Geometry: final body of the model. Coordinates: model frame, mm. Face numbers are marked on the shaded views. A direction names the side the tool comes from. Coordinates: 2 decimals unless noted, no trailing zeros. Loops run counter-clockwise (first coordinate to the right, second up) from the corner with the lowest first, then second, coordinate; pieces in that order, holes last. Notation, with made-up numbers: (5, -6.5) -> (55, -6.5) arc R18 ccw to (55, 17.5) -> close; hole circle Ø10 at (-19, 61.25). An arc over 180 degrees is marked (long way). One line per item, written item: value. Start each with the question number.
Item 1: Section query A-A on z = 0. Return loops of the section in (x, y), then the cut area to 3 significant figures.
Item 2: Contact query for flat-ended pins moving along their axis: pin 1 Ø2.5 at (x, z) = (60, 0) entering from +Y; pin 2 Ø3 at (x, z) = (45, 2) entering from -Y; pin 3 Ø1.5 at (y, z) = (1, -1.5) entering from +X. Output: stop coordinate, or through.
Item 3: Section query D-D on x = 48.5. Return loops of the section in (y, z), then the cut area to 3 significant figures.
Item 4: Section query C-C on y = 6.25. Return loops of the section in (x, z).
Item 5: Ray query, probe 1 along X at (y, z) = (2.75, 0); probe 2 along Y at (x, z) = (34, 1.15); probe 3 along X at (y, z) = (5.5, 0). Return the intervals inside material, ascending. Write a range as from..to.
Item 6: Section query B-B on y = 3.25. Return loops of the section in (x, z).
Item 7: Set-up query: the marked faces 1 and 2. Return all of +Z, -Z, +X, -X, +Y, -Y with unobstructed straight access to the full face (end or side cutting, diameter ignored); none if empty.
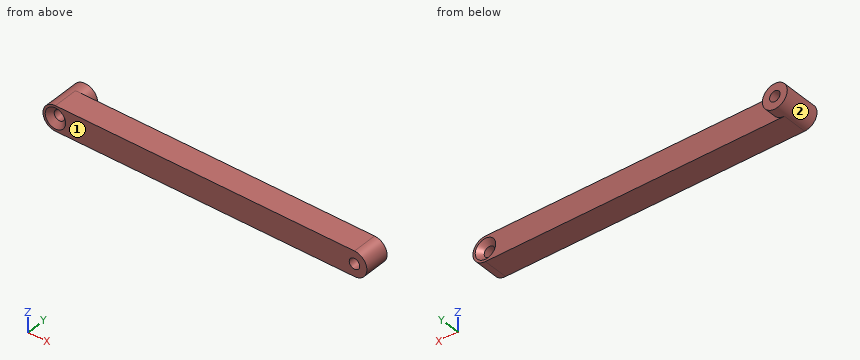
from build123d import *

# Parameters (mm, degrees)
SKETCH1_R           = 1.05
BOSS_EXTRUDE1_DEPTH = 5
CHAMFER1_SIZE       = 1
CHAMFER2_SIZE       = 1
SKETCH2_R           = 2.5
SKETCH2_R_2         = 1.05
BOSS_EXTRUDE2_DEPTH = 2.4


with BuildPart() as part:
    # Sketch1 → Boss-Extrude1 (new body)
    with BuildSketch(Plane(origin=(0, 0, 0), x_dir=(1, 0, 0), z_dir=(0, 1, 0))):
        with BuildLine():
            Line((0, 2.5), (60, 2.5))
            ThreePointArc((60, 2.5), (62.5, 0), (60, -2.5))
            Line((60, -2.5), (0, -2.5))
            ThreePointArc((0, -2.5), (-2.5, 0), (0, 2.5))
        make_face()
        with Locations(Location((0, 0, 0), (0, 0, 270))):
            Circle(SKETCH1_R, mode=Mode.SUBTRACT)
        with Locations(Location((60, 0, 0), (0, 0, 270))):
            Circle(SKETCH1_R, mode=Mode.SUBTRACT)
    extrude(amount=BOSS_EXTRUDE1_DEPTH)

    # Chamfer1
    chamfer1_edges = [part.edges().sort_by_distance(p)[0] for p in [
        (60, 5, -1.05),
    ]]
    chamfer(chamfer1_edges, length=CHAMFER1_SIZE)

    # Chamfer2
    chamfer2_edges = [part.edges().sort_by_distance(p)[0] for p in [
        (0, 0, -1.05),
    ]]
    chamfer(chamfer2_edges, length=CHAMFER2_SIZE)

    # Sketch2 → Boss-Extrude2 (add)
    with BuildSketch(Plane(origin=(0, 5, 0), x_dir=(1, 0, 0), z_dir=(0, 1, 0))):
        with Locations(Location((0, 0, 0), (0, 0, 270))):
            Circle(SKETCH2_R)
        with Locations(Location((0, 0, 0), (0, 0, 270))):
            Circle(SKETCH2_R_2, mode=Mode.SUBTRACT)
    extrude(amount=BOSS_EXTRUDE2_DEPTH)


solid = part.part
Reply:
1. outline: (-2.5, 0) -> (-2.05, 0) -> (-1.05, 1) -> (-1.05, 7.4) -> (-2.5, 7.4) -> close; (1.05, 1) -> (2.05, 0) -> (58.95, 0) -> (58.95, 4) -> (57.95, 5) -> (2.5, 5) -> (2.5, 7.4) -> (1.05, 7.4) -> close; (61.05, 0) -> (62.5, 0) -> (62.5, 5) -> (62.05, 5) -> (61.05, 4) -> close
1. area: 309 mm²
2. pin 1: stops at y = 4.2
2. pin 2: stops at y = 0
2. pin 3: stops at x = 62.38
3. outline: (0, -2.5) -> (5, -2.5) -> (5, 2.5) -> (0, 2.5) -> close
3. area: 25.0 mm²
4. outline: circle Ø5 at (0, 0); hole circle Ø2.1 at (0, 0)
5. probe 1: x = -2.5..-1.05, 1.05..58.95, 61.05..62.5
5. probe 2: y = 0..5
5. probe 3: x = -2.5..-1.05, 1.05..2.5
6. outline: (0, -2.5) -> (60, -2.5) arc R2.5 ccw to (60, 2.5) -> (0, 2.5) arc R2.5 ccw to start; hole circle Ø2.1 at (0, 0); hole circle Ø2.1 at (60, 0)
7. face 1: +Z, -Z, +X, -X, -Y
7. face 2: +Y
